from build123d import *

# Parameters (mm, degrees)
SKETCH1_R      = 3.175
EXTRUDE1_DEPTH = 171.831
SKETCH2_R      = 9.525
PISTON_DEPTH   = 2.5


with BuildPart() as part:
    # Sketch1 → Extrude1 (new body)
    with BuildSketch(Plane.XY):
        with Locations(Location((0, 0, 0), (0, 0, 180))):
            Circle(SKETCH1_R)
    extrude(amount=EXTRUDE1_DEPTH)

    # Sketch2 → Piston (add, symmetric)
    with BuildSketch(Plane.XY):
        Circle(SKETCH2_R)
    extrude(amount=PISTON_DEPTH, both=True)

    # Sketch3 → Threads (revolve, cut)
    with BuildSketch(Plane(origin=(0, 0, 0), x_dir=(0, 0, -1), z_dir=(1, 0, 0)), mode=Mode.PRIVATE) as threads_sk:
        Polygon((-171.831, 9.525), (-158.631, 9.525), (-158.631, 2.675), (-159.131, 2.675), (-159.131, 3.175), (-171.331, 3.175), (-171.831, 2.675), align=None)
    revolve(threads_sk.sketch.rotate(Axis((0, 0, 0), (0, 0, 1)), 90), axis=Axis((0, 0, 0), (0, 0, 1)), mode=Mode.SUBTRACT)


solid = part.part
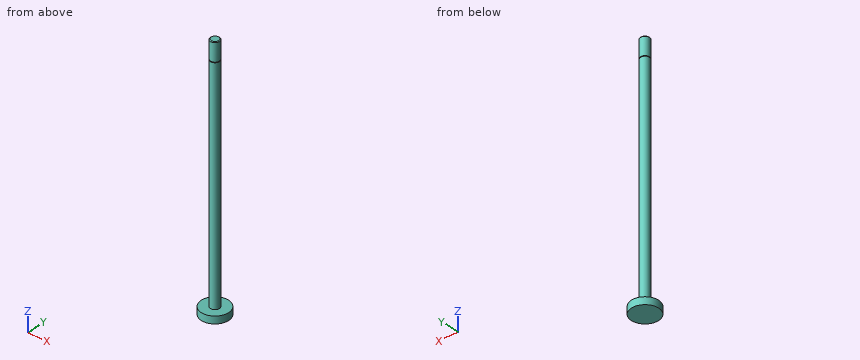
Geometry: final body of the model. Coordinates: model frame, mm. Give positions to 0.01 mm unless a question says otherwise; leave off trailing zeros. Loops run counter-clockwise (first coordinate to the right, second up) from the corner with the lowest first, then second, coordinate; pieces in that order, holes last. Notation, with made-up numbers: (32.25, -6.75) - (85.25, -6.75) arc R14 ccw to (85.25, 0.25) - close; hole circle Ø4 at (-9.5, -11). An arc over 180 degrees is marked (long way). Answer as CSV lines item,"result". Start each with the question number.
1. Pin query (flat end, axial travel): P1, Ø3, axis at x = 5, y = 2.5, coming from the +Z side; P2, Ø6, axis at y = -3.5, z = 119.5, coming from the +X side; P3, Ø3, axis at x = 1.5, z = 146.5, coming from the -Y side (3 decimals). Return the tip coordinate at first contact, or that it passes through.
2. Section C-C, the plane z = 31.5. Return loops of the section in (x, y) (3 decimals).
3. Section A-A, the plane y = 0. Return loops of the section in (x, z) (3 decimals), plus the area to 3 significant figures.
4. Ray query, L1, parallel to Z at x = 2.5, y = 2.5; L2, parallel to Z at x = -2.75, y = -1; L3, parallel to Y at x = 2.25, z = 104.5. Return the intervals inside material, ascending.
Answers:
1,P1,"stops at z = 2.5"
1,P2,"stops at x = 3.14"
1,P3,"stops at y = -3.175"
2,outline,"circle Ø6.35 at (0, 0)"
3,outline,"(-9.525, -2.5) - (9.525, -2.5) - (9.525, 2.5) - (3.175, 2.5) - (3.175, 158.631) - (2.675, 158.631) - (2.675, 159.131) - (3.175, 159.131) - (3.175, 171.331) - (2.675, 171.831) - (-2.675, 171.831) - (-3.175, 171.331) - (-3.175, 159.131) - (-2.675, 159.131) - (-2.675, 158.631) - (-3.175, 158.631) - (-3.175, 2.5) - (-9.525, 2.5) - close"
3,area,"1,170 mm2"
4,L1,"z = -2.5 to 2.5"
4,L2,"z = -2.5 to 158.63, 159.13 to 171.58"
4,L3,"y = -2.24 to 2.24"
